Verification items for the finished model (mm, model axes). Face numbers are marked on the shaded views. A direction names the side the tool comes from. Give positions to 0.01 mm unless a question says otherwise; leave off trailing zeros. Order: outer loops, then holes, each group sorted by start corner. A loop starts at its lowest first (then second) coordinate and runs counter-clockwise, first axis right, second up.
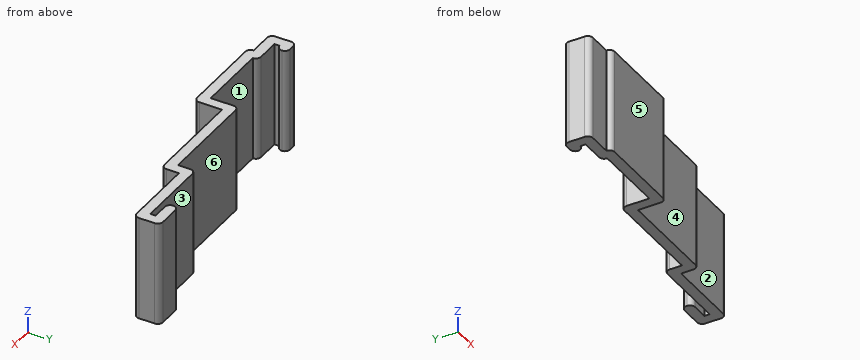
from build123d import *

# Parameters (mm, degrees)
F1_DEPTH = 30
F2_R     = 1.49999


# Not quite as in the source:
# - a fillet or chamfer is up to 0.001 mm smaller than in the source, because OpenCascade refuses the exact size


with BuildPart() as f1:
    # F0 (on Top) → F1 (new body)
    with BuildSketch(Plane.XY):
        Polygon((0, 8), (0, 0), (-20.5, 0), (-20.5, 1.5), (-28.5, 1.5), (-28.5, 3), (-27, 3), (-27, 6), (-31.5, 6), (-31.5, -1.5), (-23.5, -1.5), (-23.5, -3), (3, -3), (3, 5), (32.5, 5), (32.5, 10), (54.5, 10), (54.5, 17.5), (45.5, 17.5), (45.5, 14.5), (51.5, 14.5), (51.5, 13), (29.5, 13), (29.5, 8), align=None)
    extrude(amount=F1_DEPTH)

    # F2 (radius 1.5 in the source; OpenCascade refuses exactly that, so slightly less here)
    f2_edges = [f1.edges().sort_by_distance(p)[0] for p in [
        (-23.5, -3, 15),
        (-31.5, -1.5, 15),
        (-20.5, 1.5, 15),
        (-27, 6, 15),
        (-27, 3, 15),
        (-31.5, 6, 15),
        (3, -3, 15),
        (0, 8, 15),
        (32.5, 5, 15),
        (29.5, 13, 15),
        (45.5, 17.5, 15),
        (45.5, 14.5, 15),
        (54.5, 10, 15),
        (54.5, 17.5, 15),
    ]]
    fillet(f2_edges, radius=F2_R)


solid = f1.part
(1) Go/stop test with flat-tipped pins: pin 1 (16.5 mm diameter, centred on x = 37.5, z = 8, fed in from -Y); pin 2 (1.8 mm diameter, centred on y = 10.5, z = 10.5, fed in from -X); pin 3 (2 mm diameter, centred on y = 1, z = 9, fed in from +X). Record where each tip stops, or that it passes through.
Solved:
pin 1: stops at y = 5
pin 2: stops at x = 29.5
pin 3: stops at x = 3
(2) Section check A-A, the plane x = 41. Enter the section's corners in (y, z), then the cut area to 3 significant figures.
Solved:
outline: (10, 0) - (13, 0) - (13, 30) - (10, 30) - close
area: 90.0 mm2
(3) Scan lines: line 1 (X direction, y = 2.75, z = 7); line 2 (X direction, y = 4.5, z = 26.5); line 3 (Y direction, x = 33.5, z = 12). Record each from-to range of solid material in increasing order.
Solved:
line 1: x = -31.5 to -28.5, 0 to 3
line 2: x = -31.5 to -27, 0 to 3
line 3: y = 10 to 13
(4) Set-up check for the marked faces 4, 5 and 6: record each of +Z, -Z, +X, -X, +Y, -Y from which the full face is reachable in a straight line by a thin tool's end or side.
Solved:
face 4: +Z, -Z, +X, -Y
face 5: +Z, -Z, +X, -X, -Y
face 6: +Z, -Z, -X, +Y
(5) Release check for a two-part mould opening along Y. For the marked faces 1, 2 and 3 record: pulls with the +Y half, pulls with the -Y half, needs draft (parallel to the pull), parting line crosses it, or undercut.
Solved:
face 1: pulls with the +Y half
face 2: pulls with the -Y half
face 3: undercut
